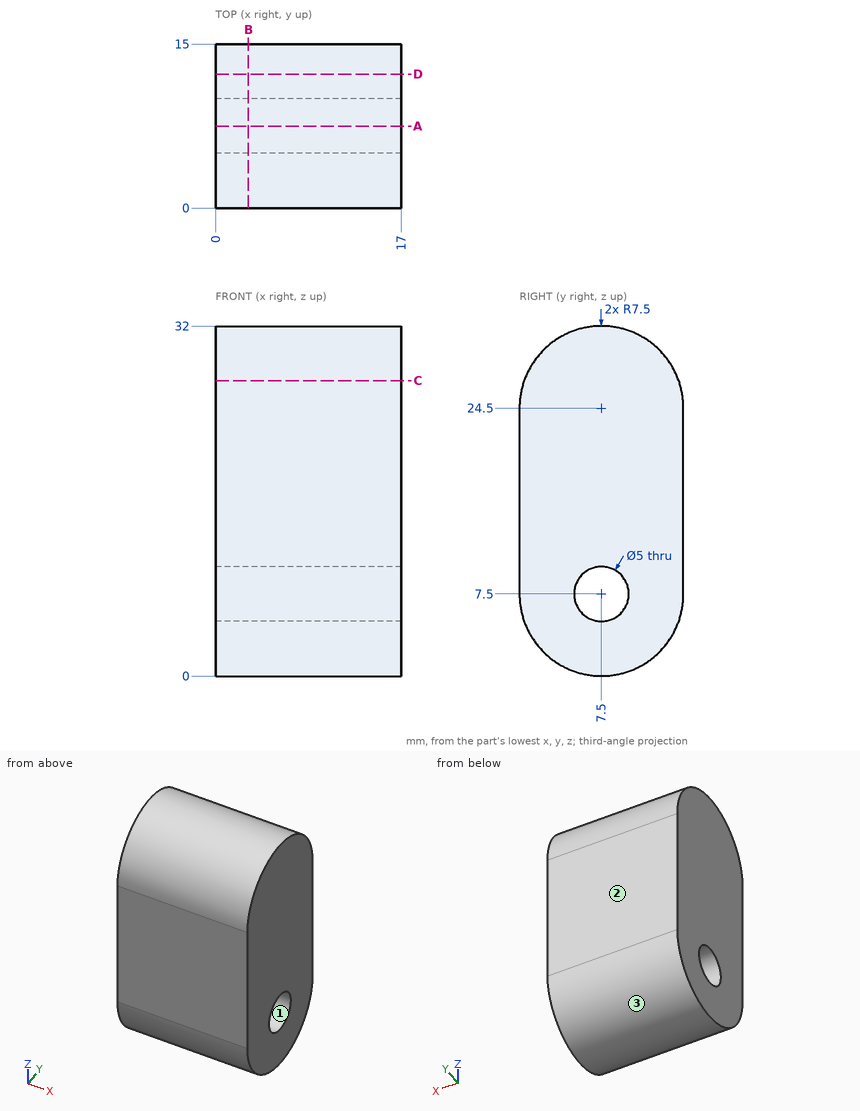
The figure shows three views and two pictorial views of one solid part (mm, origin at its lowest corner). Answer the questions. Coordinates: 2 decimals unless noted, no trailing zeros. Write each loop counter-clockwise with the first axis right and the second up, starting at its lowest first coordinate (ties: lowest second). Pieces come first, ordered by that corner, then holes. Notation, with made-up numbers: M 83.25,87 L 127.25,87 A17 cw 127.25,114 Z; hole C 75.25,60.25 d10. An arc over 180 degrees is marked long. Answer as CSV lines item,"result". Start each with the question number.
Item 1: Section D-D on y = 12.25 is taken. Write down the section's boundary in (x, z).
Item 2: Section B-B on x = 3 is taken. Write down the section's boundary in (y, z), and give its area (3 significant figures).
Item 3: Consider L1, parallel to Y at x = 6.5, z = 7.5; L2, parallel to Y at x = 2.5, z = 9.5; L3, parallel to Z at x = 2.75, y = 7.75. Determine where each line is inside the solid, lowest interval first.
Item 4: Section C-C on z = 27 is taken. Write down the section's boundary in (x, y).
Item 5: Section A-A on y = 7.5 is taken. Write down the section's boundary in (x, z).
Item 6: A flat-ended cylindrical pin translates along its axis: P1, Ø6, axis at x = 15, y = 8.5, coming from the +Z side. Find the tip coordinate at first contact, or state that the pin passes through.
Item 7: Determine the mould class of the marked faces 1, 2 and 3 for opening direction Z: released by +Z, released by -Z, zero draft, split by the parting line, or undercut.
Checks:
1,outline,"M 0,1.7 L 17,1.7 L 17,30.3 L 0,30.3 Z"
2,outline,"M 0,7.5 A7.5 ccw 15,7.5 L 15,24.5 A7.5 ccw 0,24.5 Z; hole C 7.5,7.5 d5"
2,area,"412 mm²"
3,L1,"y = 0 to 5, 10 to 15"
3,L2,"y = 0 to 6, 9 to 15"
3,L3,"z = 0 to 5.01, 9.99 to 32"
4,outline,"M 0,0.43 L 17,0.43 L 17,14.57 L 0,14.57 Z"
5,outline,"M 0,0 L 17,0 L 17,5 L 0,5 Z; M 0,10 L 17,10 L 17,32 L 0,32 Z"
6,P1,"stops at z = 32"
7,face 1,"undercut"
7,face 2,"zero draft"
7,face 3,"released by -Z"
